```python
from build123d import *

# Parameters (mm, degrees)
SKIZZE1_W                       = 10
SKIZZE1_H                       = 80
AUFSATZ_LINEAR_AUSTRAGEN1_DEPTH = 12.75
F_6_0_6_DURCHMESSER_BOHRUNG1_D  = 6


with BuildPart() as part:
    # Skizze1 → Aufsatz-Linear austragen1 (new body)
    with BuildSketch(Plane.XY):
        with Locations((-10.949316523, -25.997467638)):
            Rectangle(SKIZZE1_W, SKIZZE1_H)
    extrude(amount=AUFSATZ_LINEAR_AUSTRAGEN1_DEPTH)

    # Ø6.0 (6) Durchmesser Bohrung1 (through all)
    with Locations(Plane(origin=(-5.949316523, 0, 0), x_dir=(0, 0, -1), z_dir=(1, 0, 0))):
        with Locations((-6.375, -56.597467638)):
            Hole(F_6_0_6_DURCHMESSER_BOHRUNG1_D / 2)


solid = part.part
```
Part model, mm, in its own coordinate system. Round coordinates to 2 decimals unless told otherwise and drop trailing zeros. Write each loop counter-clockwise with the first axis right and the second up, starting at its lowest first coordinate (ties: lowest second). Pieces come first, ordered by that corner, then holes. Notation, with made-up numbers: (29, -21.5) -> (67, -21.5) arc R20 ccw to (67, 11.5) -> close; hole circle Ø5 at (-37.5, 43.5). An arc over 180 degrees is marked (long way). Return JSON: item names as keys, results as strings. Group by question number.
Q1. Saw through at A-A on z = 5.25. Write the cut outline in (x, y).
Q2. Probe L1, parallel to Y at x = -8, z = 6; L2, parallel to Z at x = -13, y = -59; L3, parallel to Y at x = -15.5, z = 4.75. List the from-to ranges inside material, lowest first. Write a range as [from, to].
Q3. Saw through at B-B on x = -12.5. Write the cut outline in (y, z) (3 decimals), plus the area to 3 significant figures.
Q4. Mould opens along Z. For faces 1 (the flat face through (-11, -25, 12.75)), 2 (the cylindrical face through (-11.02, -59.26, 7.76)), 3 (the flat face through (-11, -25, 0)), 4 (the flat face through (-11, 14.003, 6)) say: pulls with the +Z half, pulls with the -Z half, needs draft (parallel to the pull), parting line crosses it, or undercut.
Answer:
{
 "1": {"outline": "(-15.95, -66) -> (-5.95, -66) -> (-5.95, -59.38) -> (-15.95, -59.38) -> close; (-15.95, -53.82) -> (-5.95, -53.82) -> (-5.95, 14) -> (-15.95, 14) -> close"},
 "2": {"L1": "[-66, -59.57], [-53.62, 14]", "L2": "[0, 4.58], [8.17, 12.75]", "L3": "[-66, -59.12], [-54.08, 14]"},
 "3": {"outline": "(-65.997, 0) -> (14.003, 0) -> (14.003, 12.75) -> (-65.997, 12.75) -> close; hole circle Ø6 at (-56.597, 6.375)", "area": "992 mm2"},
 "4": {"face 1": "pulls with the +Z half", "face 2": "undercut", "face 3": "pulls with the -Z half", "face 4": "needs draft"}
}
